Design review of the part built by this model. Coordinates are the model's own, in mm. A direction names the side the tool comes from. Give positions to 0.01 mm unless a question says otherwise; leave off trailing zeros. Write each loop counter-clockwise with the first axis right and the second up, starting at its lowest first coordinate (ties: lowest second). Pieces come first, ordered by that corner, then holes. Notation, with made-up numbers: (30.5, 23.5) -> (48.5, 23.5) arc R13 ccw to (48.5, 38.5) -> close; hole circle Ø4 at (1, 51.25). An arc over 180 degrees is marked (long way). Answer as a JSON object with one key per item and string values.
```python
from build123d import *

# Parameters (mm, degrees)
SKETCH_1_W          = 240
SKETCH_1_H          = 260
EXTRUDE_1_DEPTH     = 4
SKETCH_2_R          = 2
CUT_EXTRUDE_1_DEPTH = 177.963273026
SKETCH_3_W          = 30
SKETCH_3_H          = 260
CUT_EXTRUDE_2_DEPTH = 6
FILLET_2_R          = 10
FILLET_3_R          = 120
SKETCH_4_R          = 83
CUT_EXTRUDE_3_DEPTH = 6
SKETCH_5_W          = 5.842752146
SKETCH_5_H          = 157.729812976
EXTRUDE_2_DEPTH     = 8
FILLET_4_R          = 2
CHAMFER_1_SIZE      = 1.5


with BuildPart() as part:
    # Эскиз1 → Бобышка-Вытянуть1 (new body)
    with BuildSketch(Plane(origin=(0, 0, 0), x_dir=(1, 0, 0), z_dir=(0, 1, 0))):
        Rectangle(SKETCH_1_W, SKETCH_1_H)
    extrude(amount=EXTRUDE_1_DEPTH)

    # Эскиз2 → Вырез-Вытянуть1 (cut, through all)
    with BuildSketch(Plane(origin=(0, 4, 0), x_dir=(1, 0, 0), z_dir=(0, 1, 0))):
        with Locations(Location((83, 122, 0), (0, 0, 270))):
            Circle(SKETCH_2_R)
        with Locations(Location((13, 122, 0), (0, 0, 270))):
            Circle(SKETCH_2_R)
        with Locations(Location((83, -122, 0), (0, 0, 90))):
            Circle(SKETCH_2_R)
        with Locations(Location((13, -122, 0), (0, 0, 90))):
            Circle(SKETCH_2_R)
        with Locations(Location((-110, 10, 0), (0, 0, 270))):
            Circle(SKETCH_2_R)
        with Locations(Location((-110, -10, 0), (0, 0, 270))):
            Circle(SKETCH_2_R)
        with Locations(Location((-85, 85, 0), (0, 0, 270))):
            Circle(SKETCH_2_R)
        with Locations(Location((85, 85, 0), (0, 0, 270))):
            Circle(SKETCH_2_R)
        with Locations(Location((-85, -85, 0), (0, 0, 270))):
            Circle(SKETCH_2_R)
        with Locations(Location((85, -85, 0), (0, 0, 270))):
            Circle(SKETCH_2_R)
    extrude(amount=-CUT_EXTRUDE_1_DEPTH, mode=Mode.SUBTRACT)

    # Эскиз3 → Вырез-Вытянуть2 (cut)
    with BuildSketch(Plane(origin=(0, 4, 0), x_dir=(1, 0, 0), z_dir=(0, 1, 0))):
        with Locations((105, 0)):
            Rectangle(SKETCH_3_W, SKETCH_3_H)
    extrude(amount=-CUT_EXTRUDE_2_DEPTH, mode=Mode.SUBTRACT)

    # Скругление2
    fillet_2_edges = [part.edges().sort_by_distance(p)[0] for p in [
        (90, 2, 130),
        (90, 2, -130),
    ]]
    fillet(fillet_2_edges, radius=FILLET_2_R)

    # Скругление3
    fillet_3_edges = [part.edges().sort_by_distance(p)[0] for p in [
        (-120, 2, 130),
        (-120, 2, -130),
    ]]
    fillet(fillet_3_edges, radius=FILLET_3_R)

    # Эскиз4 → Вырез-Вытянуть3 (cut)
    with BuildSketch(Plane(origin=(0, 4, 0), x_dir=(1, 0, 0), z_dir=(0, 1, 0))):
        with Locations(Location((0, 0, 0), (0, 0, 270))):
            Circle(SKETCH_4_R)
    extrude(amount=-CUT_EXTRUDE_3_DEPTH, mode=Mode.SUBTRACT)

    # Эскиз5 → Бобышка-Вытянуть2 (add)
    with BuildSketch(Plane(origin=(0, 4, 0), x_dir=(1, 0, 0), z_dir=(0, 1, 0))):
        with Locations((87.078623927, 0)):
            Rectangle(SKETCH_5_W, SKETCH_5_H)
    extrude(amount=EXTRUDE_2_DEPTH)

    # Скругление4
    fillet_4_edges = [part.edges().sort_by_distance(p)[0] for p in [
        (90, 12, 0),
        (87.078623927, 12, -78.864906488),
        (84.157247854, 12, 0),
        (87.078623927, 12, 78.864906488),
    ]]
    fillet(fillet_4_edges, radius=FILLET_4_R)

    # Фаска1
    chamfer_1_edges = [part.edges().sort_by_distance(p)[0] for p in [
        (90, 0, 0),
        (40, 0, -130),
        (87.071067812, 0, 127.071067812),
        (87.071067812, 0, -127.071067812),
        (-120, 0, 0),
        (40, 0, 130),
        (-84.852813742, 0, 94.852813742),
        (-84.852813742, 0, -94.852813742),
    ]]
    chamfer(chamfer_1_edges, length=CHAMFER_1_SIZE)


solid = part.part
```
(1) We need section B-B, the plane x = 30.5. State the section outline as (y, z) points, then the cut area to 3 significant figures.
Here are the results:
{"outline": "(0, -128.5) -> (1.5, -130) -> (4, -130) -> (4, -77.19) -> (0, -77.19) -> close; (0, 77.19) -> (4, 77.19) -> (4, 130) -> (1.5, 130) -> (0, 128.5) -> close", "area": "420 mm²"}
(2) We need section A-A, the plane z = 2.5. State the section outline as (x, y) points, then the cut area to 3 significant figures.
Here are the results:
{"outline": "(-120, 1.5) -> (-118.5, 0) -> (-82.96, 0) -> (-82.96, 4) -> (-120, 4) -> close; (82.96, 0) -> (88.5, 0) -> (90, 1.5) -> (90, 10) arc R2 ccw to (88, 12) -> (86.16, 12) arc R2 ccw to (84.16, 10) -> (84.16, 4) -> (82.96, 4) -> close", "area": "219 mm²"}
(3) The part is to be moulded in two halves that separate along X. For faces 4 (the cylindrical face through (24.931, 2.028, 79.167)), 5 (the flat face through (87, 7, -78.865)), 6 (the conical face through (-84.88, 0.24, 93.03)), say which applies: +X half, -X half, draft (parallel to the pull), parting line (faces both ways), or undercut.
Here are the results:
{"face 4": "undercut", "face 5": "draft", "face 6": "-X half"}
(4) Clearance check with flat-ended pins moving along their axes: pin 1 (4.5 mm diameter, centred on x = 88.5, y = 8, fed in from +Z); pin 2 (5 mm diameter, centred on x = 13, z = 122, fed in from +Y); pin 3 (6.5 mm diameter, centred on x = 86.5, y = 6, fed in from -Z). State where each tip first meets the part, or that it passes through.
Here are the results:
{"pin 1": "stops at z = 78.86", "pin 2": "stops at y = 4", "pin 3": "stops at z = -129.19"}
(5) For line 1 along X through (y, z) = (2.4, 0); line 2 along X through (y, z) = (1.5, -31); line 3 along Y through (x, z) = (-61, 76), list the stretches that pass through material, from the lowest coordinate up.
Here are the results:
{"line 1": "x = -120 to -83, 83 to 90", "line 2": "x = -118.15 to -76.99, 76.99 to 90", "line 3": "y = 0 to 4"}
(6) For faces 1 (the cylindrical face through (-85.781, 2.768, -93.915)), 2 (the flat face through (84.157, 7, 1)), 3 (the flat face through (87, 7, 78.865)), list the 3-axis set-ups (+Z, -Z, +X, -X, +Y, -Y) from which the entire face can be reached by the end or side of a thin tool; tool diameter is ignored.
Here are the results:
{"face 1": "-Z, -X, +Y, -Y", "face 2": "+Z, -Z, -X, +Y", "face 3": "+Z, +X, -X, +Y"}
(7) We need section C-C, the plane x = 68. State the section outline as (y, z) points.
Here are the results:
{"outline": "(0, -128.5) -> (1.5, -130) -> (4, -130) -> (4, -47.59) -> (0, -47.59) -> close; (0, 47.59) -> (4, 47.59) -> (4, 130) -> (1.5, 130) -> (0, 128.5) -> close"}
